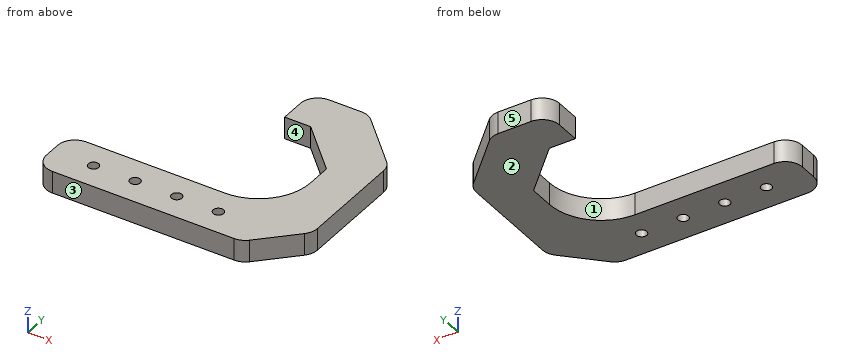
```python
from build123d import *

# Parameters (mm, degrees)
SKETCH1_W           = 60
SKETCH1_H           = 15
SKETCH1_R           = 1.5
BOSS_EXTRUDE1_DEPTH = 6.35
FILLET1_R           = 15
CHAMFER1_SIZE       = 13
FILLET3_R           = 5
CHAMFER2_SIZE       = 12.5
CHAMFER3_SIZE       = 16
FILLET4_R           = 5
FILLET5_R           = 5


with BuildPart() as part:
    # Sketch1 → Boss-Extrude1 (new body)
    with BuildSketch(Plane.XY):
        with Locations((30, 7.5)):
            Rectangle(SKETCH1_W, SKETCH1_H)
        with Locations((12, 7.5)):
            Circle(SKETCH1_R, mode=Mode.SUBTRACT)
        with Locations((24, 7.5)):
            Circle(SKETCH1_R, mode=Mode.SUBTRACT)
        with Locations((36, 7.5)):
            Circle(SKETCH1_R, mode=Mode.SUBTRACT)
        with Locations((48, 7.5)):
            Circle(SKETCH1_R, mode=Mode.SUBTRACT)
        Polygon((60, 15), (60, 0), (72, 0), (72, 50), (60, 50), align=None)
        Polygon((39.5, 50), (60, 50), (72, 50), (72, 62), (39.5, 62), align=None)
    extrude(amount=BOSS_EXTRUDE1_DEPTH)

    # Fillet1
    fillet1_edges = [part.edges().sort_by_distance(p)[0] for p in [
        (60, 15, 3.175),
    ]]
    fillet(fillet1_edges, radius=FILLET1_R)

    # Chamfer1
    chamfer1_edges = [part.edges().sort_by_distance(p)[0] for p in [
        (60, 50, 3.175),
    ]]
    chamfer(chamfer1_edges, length=CHAMFER1_SIZE)

    # Fillet3
    fillet3_edges = [part.edges().sort_by_distance(p)[0] for p in [
        (39.5, 62, 3.175),
    ]]
    fillet(fillet3_edges, radius=FILLET3_R)

    # Chamfer2
    chamfer2_edges = [part.edges().sort_by_distance(p)[0] for p in [
        (72, 0, 3.175),
    ]]
    chamfer(chamfer2_edges, length=CHAMFER2_SIZE)

    # Chamfer3
    chamfer3_edges = [part.edges().sort_by_distance(p)[0] for p in [
        (72, 62, 3.175),
    ]]
    chamfer(chamfer3_edges, length=CHAMFER3_SIZE)

    # Fillet4
    fillet4_edges = [part.edges().sort_by_distance(p)[0] for p in [
        (72, 12.5, 3.175),
        (59.5, 0, 3.175),
        (56, 62, 3.175),
        (72, 46, 3.175),
    ]]
    fillet(fillet4_edges, radius=FILLET4_R)

    # Fillet5
    fillet5_edges = [part.edges().sort_by_distance(p)[0] for p in [
        (0, 0, 3.175),
        (0, 15, 3.175),
    ]]
    fillet(fillet5_edges, radius=FILLET5_R)


solid = part.part
```
Geometry check sheet. Reference: the model listing, model coordinates, mm. Face numbers are marked on the shaded views. A direction names the side the tool comes from. Give positions to 0.01 mm unless a question says otherwise; leave off trailing zeros. Write each loop counter-clockwise with the first axis right and the second up, starting at its lowest first coordinate (ties: lowest second). Pieces come first, ordered by that corner, then holes.
1) Section check B-B, the plane z = 4.5. Record the boundary of the cut face in (x, y).
2) Gauge pin test, flat end, axial feed: pin 1 (3 mm diameter, centred on y = 32, z = 2.5, fed in from -X). Record the tip position at first contact, or that the pin passes through.
3) Section check A-A, the plane x = 24. Record the boundary of the cut face in (y, z).
4) Access from +Z, -Z, +X, -X, +Y, -Y to the whole of each face (thin tool, end or side, straight path). Record for the marked faces 4 and 5.
5) Section check D-D, the plane x = 55. Record the boundary of the cut face in (y, z), and give its area (3 significant figures).
6) Section check C-C, the plane y = 7.5. Record the boundary of the cut face in (x, z).
7) Material ranges on L1, parallel to Y at x = 48, z = 4.5; L2, parallel to Y at x = 12, z = 2; L3, parallel to Y at x = 28, z = 0.75, recorded low to high.
8) Release check for a two-part mould opening along Y. For the marked faces 1, 2 and 3 record: pulls with the +Y half, pulls with the -Y half, needs draft (parallel to the pull), parting line crosses it, or undercut.
Computed:
1. outline: (0, 5) arc R5 ccw to (5, 0) - (57.43, 0) arc R5 ccw to (60.96, 1.46) - (70.54, 11.04) arc R5 ccw to (72, 14.57) - (72, 43.93) arc R5 ccw to (70.54, 47.46) - (57.46, 60.54) arc R5 ccw to (53.93, 62) - (44.5, 62) arc R5 ccw to (39.5, 57) - (39.5, 50) - (47, 50) - (60, 37) - (60, 30) arc R15 cw to (45, 15) - (5, 15) arc R5 ccw to (0, 10) - close; hole circle Ø3 at (12, 7.5); hole circle Ø3 at (24, 7.5); hole circle Ø3 at (36, 7.5); hole circle Ø3 at (48, 7.5)
2. pin 1: stops at x = 60
3. outline: (0, 0) - (6, 0) - (6, 6.35) - (0, 6.35) - close; (9, 0) - (15, 0) - (15, 6.35) - (9, 6.35) - close
4. face 4: +Z, -Z, -X
4. face 5: +Z, -Z, +X, -X, +Y
5. outline: (0, 0) - (18.82, 0) - (18.82, 6.35) - (0, 6.35) - close; (42, 0) - (61.88, 0) - (61.88, 6.35) - (42, 6.35) - close
5. area: 246 mm2
6. outline: (0, 0) - (10.5, 0) - (10.5, 6.35) - (0, 6.35) - close; (13.5, 0) - (22.5, 0) - (22.5, 6.35) - (13.5, 6.35) - close; (25.5, 0) - (34.5, 0) - (34.5, 6.35) - (25.5, 6.35) - close; (37.5, 0) - (46.5, 0) - (46.5, 6.35) - (37.5, 6.35) - close; (49.5, 0) - (67, 0) - (67, 6.35) - (49.5, 6.35) - close
7. L1: y = 0 to 6, 9 to 15.3, 49 to 62
7. L2: y = 0 to 6, 9 to 15
7. L3: y = 0 to 15
8. face 1: undercut
8. face 2: needs draft
8. face 3: pulls with the -Y half
